```python
from build123d import *

# Parameters (mm, degrees)
F1_DEPTH = 15
F2_R     = 3
F3_R     = 1


with BuildPart() as f1:
    # F0 (on Top) → F1 (new body)
    with BuildSketch(Plane.XY):
        with BuildLine():
            Line((150, 15), (52.915026, 15))
            ThreePointArc((52.915026, 15), (-55, 0), (52.915026, -15))
            Line((52.915026, -15), (150, -15))
            Line((150, -15), (150, 15))
        make_face()
        with BuildLine():
            ThreePointArc((-21.25, -36.80608), (-30.052038, -30.052038), (-36.80608, -21.25))
            Line((-36.80608, -21.25), (-41.136207, -23.75))
            ThreePointArc((-41.136207, -23.75), (-45.881477, 12.293905), (-23.75, 41.136207))
            Line((-23.75, 41.136207), (-21.25, 36.80608))
            ThreePointArc((-21.25, 36.80608), (-10.999809, 41.051848), (0, 42.5))
            Line((0, 42.5), (0, 47.5))
            ThreePointArc((0, 47.5), (33.587572, 33.587572), (47.5, 0))
            Line((47.5, 0), (42.5, 0))
            ThreePointArc((42.5, 0), (41.051848, -10.999809), (36.80608, -21.25))
            Line((36.80608, -21.25), (41.136207, -23.75))
            ThreePointArc((41.136207, -23.75), (12.293905, -45.881477), (-23.75, -41.136207))
            Line((-23.75, -41.136207), (-21.25, -36.80608))
        make_face(mode=Mode.SUBTRACT)
    extrude(amount=F1_DEPTH)

    # F2
    f2_edges = [f1.edges().sort_by_distance(p)[0] for p in [
        (101.457513, 15, 15),
        (150, 0, 15),
        (101.457513, -15, 15),
        (-55, 0, 15),
        (101.457513, -15, 0),
        (150, 0, 0),
        (-55, 0, 0),
        (101.457513, 15, 0),
    ]]
    fillet(f2_edges, radius=F2_R)

    # F3
    f3_edges = [f1.edges().sort_by_distance(p)[0] for p in [
        (36.80608, -21.25, 7.5),
        (42.5, 0, 7.5),
        (0, 42.5, 7.5),
        (-21.25, 36.80608, 7.5),
        (-21.25, -36.80608, 7.5),
        (-36.80608, -21.25, 7.5),
    ]]
    fillet(f3_edges, radius=F3_R)


solid = f1.part
```
CAD build for the part. Positions are in the model's coordinates, mm. A direction names the side the tool comes from. Round coordinates to 2 decimals unless told otherwise and drop trailing zeros. Write each loop counter-clockwise with the first axis right and the second up, starting at its lowest first coordinate (ties: lowest second). Pieces come first, ordered by that corner, then holes. Notation, with made-up numbers: (-28.5, 42.25) -> (-19.5, 42.25) arc R28 cw to (-19.5, 63.25) -> close; hole circle Ø1 at (4, 10). An arc over 180 degrees is marked (long way). Answer in a Markdown table with one row per item. Add a question column.
Item 1: Saw through at B-B, the plane x = 111. Write the cut outline in (y, z), then the cut area to 3 significant figures.
Item 2: Mould opens along Y. For faces 1 (the face through (150, 0, 7)), 2 (the face through (-11.137, 41.015, 7.395)), 3 (the face through (-29.951, -30.152, 7.395)), 4 (the face through (-54.956, 2.206, 7.437)) say: pulls with the +Y half, pulls with the -Y half, needs draft (parallel to the pull), parting line crosses it, or undercut.
Item 3: Which spindle directions (+Z, -Z, +X, -X, +Y, -Y) get a long thin tool onto all of the face, cutting with end or side? Do faces 5 (the face through (0, 45, 7)), 6 (the face through (102, 15, 7)), 7 (the face through (101, -15, 7)). Say none if no direction does.
Item 4: Saw through at A-A, the plane z = 5.75. Write the cut outline in (x, y), then the cut area to 3 significant figures.
Item 5: Drill centre lines: line 1 (X direction, y = 0.5, z = 9.5); line 2 (X direction, y = -40, z = 2); line 3 (Y direction, x = 138, z = 5). Where is each one in solid material? Low to high. Write a range as from..to.
Item 6: Drop flat-ended pins along their axis: pin 1 Ø2 at (x, z) = (124.5, 4.5) entering from -Y; pin 2 Ø8 at (x, y) = (41.5, -41) entering from +Z; pin 3 Ø1.2 at (x, z) = (45.5, 4) entering from +Y. Give the stop position or say it passes through.
Findings below:
| question | item | result |
|---|---|---|
| 1 | outline | (-15, 3) arc R3 ccw to (-12, 0) -> (12, 0) arc R3 ccw to (15, 3) -> (15, 12) arc R3 ccw to (12, 15) -> (-12, 15) arc R3 ccw to (-15, 12) -> close |
| 1 | area | 442 mm^2 |
| 2 | face 1 | needs draft |
| 2 | face 2 | undercut |
| 2 | face 3 | undercut |
| 2 | face 4 | parting line crosses it |
| 3 | face 5 | +Z, -Z |
| 3 | face 6 | +Z, -Z, +X, +Y |
| 3 | face 7 | +Z, -Z, +X, -Y |
| 4 | outline | (52.92, -15) -> (150, -15) -> (150, 15) -> (52.92, 15) arc R55 ccw (long way) to start; hole (-41.14, -23.75) -> (-37.66, -21.74) arc R1 cw to (-36.31, -22.09) arc R42.5 ccw to (-22.09, -36.31) arc R1 cw to (-21.74, -37.66) -> (-23.75, -41.14) arc R47.5 ccw to (41.14, -23.75) -> (37.66, -21.74) arc R1 cw to (37.28, -20.4) arc R42.5 ccw to (42.49, -0.98) arc R1 cw to (43.49, 0) -> (47.5, 0) arc R47.5 ccw to (0, 47.5) -> (0, 43.49) arc R1 cw to (-0.98, 42.49) arc R42.5 ccw to (-20.4, 37.28) arc R1 cw to (-21.74, 37.66) -> (-23.75, 41.14) arc R47.5 ccw to start |
| 4 | area | 5,640 mm^2 |
| 5 | line 1 | x = -55..-47.5, 47.5..150 |
| 5 | line 2 | x = -37.5..-23.09, 25.62..37.5 |
| 5 | line 3 | y = -15..15 |
| 6 | pin 1 | stops at y = -15 |
| 6 | pin 2 | stops at z = 13.88 |
| 6 | pin 3 | stops at y = 31.76 |
